Geometry check sheet. Reference: the model listing, model coordinates, mm. Face numbers are marked on the shaded views. A direction names the side the tool comes from. Give positions to 0.01 mm unless a question says otherwise; leave off trailing zeros. Loops run counter-clockwise (first coordinate to the right, second up) from the corner with the lowest first, then second, coordinate; pieces in that order, holes last. Notation, with made-up numbers: (54, -32) -> (61, -32) arc R27 ccw to (61, -11) -> close; hole circle Ø2 at (78, 75.25). An arc over 180 degrees is marked (long way). One line per item, written item: value. Start each with the question number.
(1) Sectioned sample at A-A, the plane y = 7.25. Record the cut outline in (x, z), then the cut area to 3 significant figures.
(2) Draft check along Z on the marked faces 4, 5 and 6. Enter one of: pulls with the +Z half, pulls with the -Z half, needs draft (parallel to the pull), parting line crosses it, or undercut.
(3) Gauge pin test, flat ends, axial feed: pin 1 Ø1.8 at (x, z) = (12.73, 12.73) entering from -Y; pin 2 Ø5 at (x, z) = (-12.73, -12.73) entering from +Y; pin 3 Ø10 at (x, z) = (-7, -18) entering from +Y. Record the tip position at first contact, or that the pin passes through.
(4) Sectioned sample at C-C, the plane x = -22. Record the cut outline in (y, z), then the cut area to 3 significant figures.
(5) Sectioned sample at D-D, the plane z = -22. Record the cut outline in (x, y), then the cut area to 3 significant figures.
(6) Scan lines: line 1 along X through (y, z) = (5, 0); line 2 along Z through (x, y) = (12, -2.5); line 3 along Y through (x, z) = (-18.5, 4.5). Record each from-to range of solid material in increasing order. Write a range as from..to.
(7) Tool access check on the marked faces 1, 2 and 3. Record the directions out of +Z, -Z, +X, -X, +Y, -Y that give a thin tool (end or side, any length) a straight path to the whole face; none if there is none.
(8) Sectioned sample at B-B, the plane y = 16. Record the cut outline in (x, z).
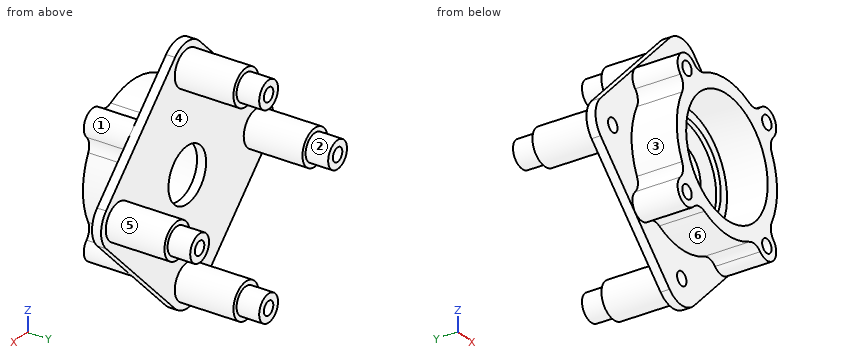
from build123d import *

# Parameters (mm, degrees)
SKETCH2_R           = 1.5
BOSS_EXTRUDE1_DEPTH = 2
SKETCH2_4_R         = 4
SKETCH2_4_R_2       = 1.5
BOSS_EXTRUDE2_DEPTH = 20
CUT_EXTRUDE1_START  = 20
SKETCH2_5_R         = 4
SKETCH2_5_R_2       = 3
CUT_EXTRUDE1_DEPTH  = 5
SKETCH5_R           = 13
SKETCH5_R_2         = 1.5
BOSS_EXTRUDE3_DEPTH = 10
SKETCH5_3_R         = 13
SKETCH5_3_R_2       = 11
BOSS_EXTRUDE4_DEPTH = 1
SKETCH5_4_R         = 6
CUT_EXTRUDE2_DEPTH  = 10


with BuildPart() as part:
    # Sketch2 → Boss-Extrude1 (new body)
    with BuildSketch(Plane(origin=(0, 0, 0), x_dir=(1, 0, 0), z_dir=(0, 1, 0))):
        with BuildLine():
            Line((25.889087297, 3.889087297), (3.889087297, 25.889087297))
            ThreePointArc((3.889087297, 25.889087297), (0, 27.5), (-3.889087297, 25.889087297))
            Line((-3.889087297, 25.889087297), (-25.889087297, 3.889087297))
            ThreePointArc((-25.889087297, 3.889087297), (-27.5, 0), (-25.889087297, -3.889087297))
            Line((-25.889087297, -3.889087297), (-3.889087297, -25.889087297))
            ThreePointArc((-3.889087297, -25.889087297), (0, -27.5), (3.889087297, -25.889087297))
            Line((3.889087297, -25.889087297), (25.889087297, -3.889087297))
            ThreePointArc((25.889087297, -3.889087297), (27.5, 0), (25.889087297, 3.889087297))
        make_face()
        with Locations(Location((-22, 0, 0), (0, 0, 270))):
            Circle(SKETCH2_R, mode=Mode.SUBTRACT)
        with Locations(Location((0, -22, 0), (0, 0, 270))):
            Circle(SKETCH2_R, mode=Mode.SUBTRACT)
        with Locations(Location((22, 0, 0), (0, 0, 270))):
            Circle(SKETCH2_R, mode=Mode.SUBTRACT)
        with Locations(Location((0, 22, 0), (0, 0, 270))):
            Circle(SKETCH2_R, mode=Mode.SUBTRACT)
    extrude(amount=BOSS_EXTRUDE1_DEPTH)

    # Sketch2<4> → Boss-Extrude2 (add)
    with BuildSketch(Plane(origin=(0, 0, 0), x_dir=(1, 0, 0), z_dir=(0, 1, 0))):
        with Locations(Location((22, 0, 0), (0, 0, 270))):
            Circle(SKETCH2_4_R)
        with Locations(Location((22, 0, 0), (0, 0, 270))):
            Circle(SKETCH2_4_R_2, mode=Mode.SUBTRACT)
        with Locations(Location((0, -22, 0), (0, 0, 270))):
            Circle(SKETCH2_4_R)
        with Locations(Location((0, -22, 0), (0, 0, 270))):
            Circle(SKETCH2_4_R_2, mode=Mode.SUBTRACT)
        with Locations(Location((-22, 0, 0), (0, 0, 270))):
            Circle(SKETCH2_4_R)
        with Locations(Location((-22, 0, 0), (0, 0, 270))):
            Circle(SKETCH2_4_R_2, mode=Mode.SUBTRACT)
        with Locations(Location((0, 22, 0), (0, 0, 270))):
            Circle(SKETCH2_4_R)
        with Locations(Location((0, 22, 0), (0, 0, 270))):
            Circle(SKETCH2_4_R_2, mode=Mode.SUBTRACT)
    extrude(amount=BOSS_EXTRUDE2_DEPTH)

    # Sketch2<5> → Cut-Extrude1 (cut)
    with BuildSketch(Plane(origin=(0, 0, 0), x_dir=(1, 0, 0), z_dir=(0, 1, 0)).offset(CUT_EXTRUDE1_START)):
        with Locations(Location((-22, 0, 0), (0, 0, 270))):
            Circle(SKETCH2_5_R)
        with Locations(Location((-22, 0, 0), (0, 0, 270))):
            Circle(SKETCH2_5_R_2, mode=Mode.SUBTRACT)
        with Locations(Location((0, 22, 0), (0, 0, 270))):
            Circle(SKETCH2_5_R)
        with Locations(Location((0, 22, 0), (0, 0, 270))):
            Circle(SKETCH2_5_R_2, mode=Mode.SUBTRACT)
        with BuildLine():
            ThreePointArc((19, 0), (22, 3), (25, 0))
            Line((25, 0), (26, 0))
            ThreePointArc((26, 0), (22, 4), (18, 0))
            Line((18, 0), (19, 0))
        make_face()
        with BuildLine():
            Line((26, 0), (25, 0))
            ThreePointArc((25, 0), (22, -3), (19, 0))
            Line((19, 0), (18, 0))
            ThreePointArc((18, 0), (22, -4), (26, 0))
        make_face()
        with Locations(Location((0, -22, 0), (0, 0, 270))):
            Circle(SKETCH2_5_R)
        with Locations(Location((0, -22, 0), (0, 0, 270))):
            Circle(SKETCH2_5_R_2, mode=Mode.SUBTRACT)
    extrude(amount=-CUT_EXTRUDE1_DEPTH, mode=Mode.SUBTRACT)

    # Sketch5 → Boss-Extrude3 (add)
    with BuildSketch(Plane.XZ):
        with BuildLine():
            ThreePointArc((14.297039341, 7.182942718), (14.019613784, 8.984050781), (14.849242405, 10.606601718))
            ThreePointArc((14.849242405, 10.606601718), (14.849242405, 14.849242405), (10.606601718, 14.849242405))
            ThreePointArc((10.606601718, 14.849242405), (8.984050781, 14.019613784), (7.182942718, 14.297039341))
            ThreePointArc((7.182942718, 14.297039341), (0, 16), (-7.182942718, 14.297039341))
            ThreePointArc((-7.182942718, 14.297039341), (-8.984050781, 14.019613784), (-10.606601718, 14.849242405))
            ThreePointArc((-10.606601718, 14.849242405), (-14.849242405, 14.849242405), (-14.849242405, 10.606601718))
            ThreePointArc((-14.849242405, 10.606601718), (-14.019613784, 8.984050781), (-14.297039341, 7.182942718))
            ThreePointArc((-14.297039341, 7.182942718), (-16, 0), (-14.297039341, -7.182942718))
            ThreePointArc((-14.297039341, -7.182942718), (-14.019613784, -8.984050781), (-14.849242405, -10.606601718))
            ThreePointArc((-14.849242405, -10.606601718), (-14.849242405, -14.849242405), (-10.606601718, -14.849242405))
            ThreePointArc((-10.606601718, -14.849242405), (-8.984050781, -14.019613784), (-7.182942718, -14.297039341))
            ThreePointArc((-7.182942718, -14.297039341), (0, -16), (7.182942718, -14.297039341))
            ThreePointArc((7.182942718, -14.297039341), (8.984050781, -14.019613784), (10.606601718, -14.849242405))
            ThreePointArc((10.606601718, -14.849242405), (14.849242405, -14.849242405), (14.849242405, -10.606601718))
            ThreePointArc((14.849242405, -10.606601718), (14.019613784, -8.984050781), (14.297039341, -7.182942718))
            ThreePointArc((14.297039341, -7.182942718), (16, 0), (14.297039341, 7.182942718))
        make_face()
        with Locations(Location((0, 0, 0), (0, 0, 270))):
            Circle(SKETCH5_R, mode=Mode.SUBTRACT)
        with Locations(Location((12.727922061, 12.727922061, 0), (0, 0, 270))):
            Circle(SKETCH5_R_2, mode=Mode.SUBTRACT)
        with Locations(Location((12.727922061, -12.727922061, 0), (0, 0, 270))):
            Circle(SKETCH5_R_2, mode=Mode.SUBTRACT)
        with Locations(Location((-12.727922061, 12.727922061, 0), (0, 0, 270))):
            Circle(SKETCH5_R_2, mode=Mode.SUBTRACT)
        with Locations(Location((-12.727922061, -12.727922061, 0), (0, 0, 270))):
            Circle(SKETCH5_R_2, mode=Mode.SUBTRACT)
    extrude(amount=BOSS_EXTRUDE3_DEPTH)

    # Sketch5<3> → Boss-Extrude4 (add)
    with BuildSketch(Plane.XZ):
        with Locations(Location((0, 0, 0), (0, 0, 270))):
            Circle(SKETCH5_3_R)
        with Locations(Location((0, 0, 0), (0, 0, 270))):
            Circle(SKETCH5_3_R_2, mode=Mode.SUBTRACT)
    extrude(amount=BOSS_EXTRUDE4_DEPTH)

    # Sketch5<4> → Cut-Extrude2 (cut)
    with BuildSketch(Plane.XZ):
        with Locations(Location((0, 0, 0), (0, 0, 270))):
            Circle(SKETCH5_4_R)
    extrude(amount=-CUT_EXTRUDE2_DEPTH, mode=Mode.SUBTRACT)


solid = part.part
Calculated:
1. outline: circle Ø8 at (-22, 0); circle Ø8 at (0, -22); circle Ø8 at (0, 22); circle Ø8 at (22, 0); hole circle Ø3 at (-22, 0); hole circle Ø3 at (0, -22); hole circle Ø3 at (0, 22); hole circle Ø3 at (22, 0)
1. area: 173 mm2
2. face 4: undercut
2. face 5: parting line crosses it
2. face 6: pulls with the -Z half
3. pin 1: stops at y = 0
3. pin 2: stops at y = 2
3. pin 3: stops at y = 15
4. outline: (0, -7.78) -> (2, -7.78) -> (2, -4) -> (15, -4) -> (15, -3) -> (20, -3) -> (20, -1.5) -> (0, -1.5) -> close; (0, 1.5) -> (20, 1.5) -> (20, 3) -> (15, 3) -> (15, 4) -> (2, 4) -> (2, 7.78) -> (0, 7.78) -> close
4. area: 105 mm2
5. outline: (-7.78, 0) -> (-1.5, 0) -> (-1.5, 20) -> (-3, 20) -> (-3, 15) -> (-4, 15) -> (-4, 2) -> (-7.78, 2) -> close; (1.5, 0) -> (7.78, 0) -> (7.78, 2) -> (4, 2) -> (4, 15) -> (3, 15) -> (3, 20) -> (1.5, 20) -> close
5. area: 105 mm2
6. line 1: x = -26..-23.5, -20.5..-18, 18..20.5, 23.5..26
6. line 2: z = -15.64..-14.04, -11.42..-5, 5..11.42, 14.04..15.64
6. line 3: y = 0..2
7. face 1: -Y
7. face 2: +Y
7. face 3: -X, -Y
8. outline: circle Ø6 at (-22, 0); circle Ø6 at (0, -22); circle Ø6 at (0, 22); circle Ø6 at (22, 0); hole circle Ø3 at (-22, 0); hole circle Ø3 at (0, -22); hole circle Ø3 at (0, 22); hole circle Ø3 at (22, 0)
